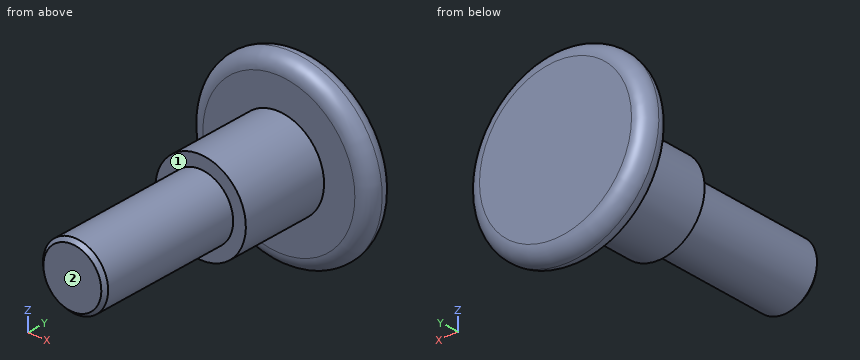
from build123d import *

# Parameters (mm, degrees)
FILETE1_R     = 2
CHANFRO1_SIZE = 0.5


with BuildPart() as part:
    # Esboço1 → Revolução1 (revolve)
    with BuildSketch(Plane.XY, mode=Mode.PRIVATE) as revolu_o1_sk:
        Polygon((0, 63.957087486), (12.5, 63.957087486), (12.5, 59.957087486), (6.25, 59.957087486), (6.25, 47.757087486), (4.5, 47.757087486), (4.5, 27.757087486), (0, 27.757087486), align=None)
    revolve(revolu_o1_sk.sketch.rotate(Axis((0, -74.716223699, 0), (0, 1, 0)), 90), axis=Axis((0, -74.716223699, 0), (0, 1, 0)))

    # Filete1
    filete1_edges = [part.edges().sort_by_distance(p)[0] for p in [
        (0, 59.957087486, 12.5),
        (0, 63.957087486, 12.5),
    ]]
    fillet(filete1_edges, radius=FILETE1_R - 0.0001)  # a hair under: the kernel refuses the full size

    # Chanfro1
    chanfro1_edges = [part.edges().sort_by_distance(p)[0] for p in [
        (0, 27.757087486, 4.5),
    ]]
    chamfer(chanfro1_edges, length=CHANFRO1_SIZE)


solid = part.part
Here's how the part is built. I have some questions about the finished solid (model axes, mm). Face numbers are marked on the shaded views. A direction names the side the tool comes from. Coordinates: 2 decimals unless noted, no trailing zeros. Order: outer loops, then holes, each group sorted by start corner. A loop starts at its lowest first (then second) coordinate and runs counter-clockwise, first axis right, second up.
Item 1: For P1, Ø5, axis at y = 40.5, z = 8, coming from the +X side; P2, Ø6, axis at x = -2, z = -7.5, coming from the -Y side; P3, Ø1, axis at x = 4, y = 53, coming from the +Z side; P4, Ø6, axis at y = 52, z = -6, coming from the -X side, each with a flat end and sliding along its axis, tell me the tip position at first contact or that it passes through.
Result sheet:
P1: passes through
P2: stops at y = 47.76
P3: stops at z = 5.18
P4: stops at x = -5.48
Item 2: For the marked faces 1 and 2, which set-ups out of +Z, -Z, +X, -X, +Y, -Y let a thin tool reach every point of the face, with its end or its side?
Result sheet:
face 1: -Y
face 2: +Z, -Z, +X, -X, -Y
Item 3: If we section it at C-C on y = 45: List the corners of the cut face in (x, z) for me.
Result sheet:
outline: circle Ø9 at (0, 0)
Item 4: I need wall thicknesses on line 1 (X direction, y = 50.5, z = 0.25) (3 decimals); line 2 (Y direction, x = 2.5, z = -9.5); line 3 (Y direction, x = 5.25, z = -0.5). Which ranges of each line are inside material? Lowest first, please.
Result sheet:
line 1: x = -6.245 to 6.245
line 2: y = 59.96 to 63.96
line 3: y = 47.76 to 63.96
